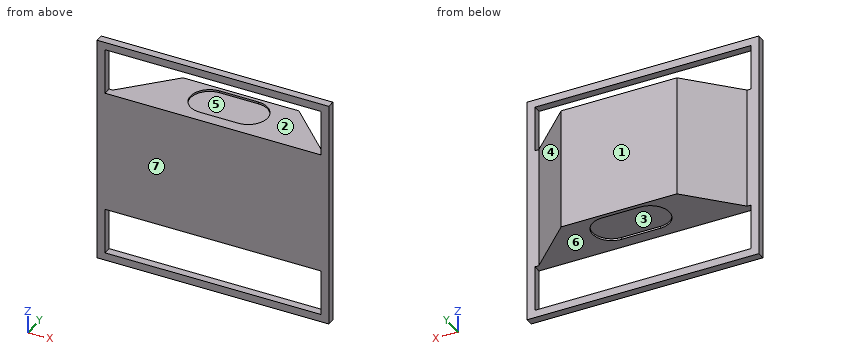
from build123d import *

# Parameters (mm, degrees)
SKETCH_1_W          = 600
SKETCH_1_H          = 600
SKETCH_1_W_2        = 560
SKETCH_1_H_2        = 120
EXTRUDE_1_DEPTH     = 20
EXTRUDE_2_DEPTH     = 320
CUT_EXTRUDE_1_DEPTH = 5
CUT_EXTRUDE_START   = -320
CUT_EXTRUDE_3_DEPTH = 5


with BuildPart() as part:
    # 草图1 → 凸台-拉伸1 (new body)
    with BuildSketch(Plane(origin=(0, 0, 0), x_dir=(1, 0, 0), z_dir=(0, 1, 0))):
        Rectangle(SKETCH_1_W, SKETCH_1_H)
        with Locations((0, 220)):
            Rectangle(SKETCH_1_W_2, SKETCH_1_H_2, mode=Mode.SUBTRACT)
        with Locations((0, -220)):
            Rectangle(SKETCH_1_W_2, SKETCH_1_H_2, mode=Mode.SUBTRACT)
    extrude(amount=EXTRUDE_1_DEPTH)

    # 草图2 → 凸台-拉伸2 (add)
    with BuildSketch(Plane.XY.offset(160)):
        Polygon((-270, 20), (-270, 0), (270, 0), (270, 20), (150, 140), (-150, 140), align=None)
    extrude(amount=-EXTRUDE_2_DEPTH)

    # 草图3 → 切除-拉伸1 (cut)
    with BuildSketch(Plane.XY.offset(160)):
        with BuildLine():
            Line((50, 130), (-50, 130))
            ThreePointArc((-50, 130), (-100, 80), (-50, 30))
            Line((-50, 30), (50, 30))
            ThreePointArc((50, 30), (100, 80), (50, 130))
        make_face()
    extrude(amount=-CUT_EXTRUDE_1_DEPTH, mode=Mode.SUBTRACT)

    # 草图3<3> → 切除-拉伸3 (cut)
    with BuildSketch(Plane.XY.offset(160).offset(CUT_EXTRUDE_START)):
        with BuildLine():
            Line((50, 130), (-50, 130))
            ThreePointArc((-50, 130), (-100, 80), (-50, 30))
            Line((-50, 30), (50, 30))
            ThreePointArc((50, 30), (100, 80), (50, 130))
        make_face()
    extrude(amount=CUT_EXTRUDE_3_DEPTH, mode=Mode.SUBTRACT)


solid = part.part
Model file for the job. Use its own axes, mm. Face numbers are marked on the shaded views. A direction names the side the tool comes from. Coordinates: 2 decimals unless noted, no trailing zeros. Loops run counter-clockwise (first coordinate to the right, second up) from the corner with the lowest first, then second, coordinate; pieces in that order, holes last. Notation, with made-up numbers: (20, 28.5) -> (70, 28.5) arc R30 ccw to (70, 56.5) -> close; hole circle Ø1 at (75.25, 85.5). An arc over 180 degrees is marked (long way). Use one line per item in the form item = value. Start each with the question number.
(1) Cut at A-A on x = 177. Give the cut face in (y, z), and give its area (3 significant figures).
(2) Cut at B-B on z = -218. Give the cut face in (x, y).
(3) Pull direction X, two halves, no side cores. Call the marked faces 1, 2, 3 and 4: pulls with the +X half, pulls with the -X half, needs draft (parallel to the pull), parting line crosses it, or undercut.
(4) Tool access for the marked faces 5, 6 and 7: list every direction of +Z, -Z, +X, -X, +Y, -Y with a clear straight run to the whole face (end or side of a thin tool).
(5) Cut at C-C on z = -48.5. Give the cut face in (x, y).
(6) Cut at D-D on x = -252. Give the cut face in (y, z), and give its area (3 significant figures).
(7) Probe probe 1 along Z at (x, y) = (-1.5, 8.5); probe 2 along Z at (x, y) = (-113.5, 58); probe 3 along Z at (x, y) = (-80, 77.5). List the from-to ranges inside material, lowest first. Write a range as from..to.
(8) Flat gauge pins, fed straight in: pin 1 (12 mm diameter, centred on x = -175.5, z = 38, fed in from +Y); pin 2 (5 mm diameter, centred on x = -191, z = 68, fed in from +Y); pin 3 (12 mm diameter, centred on x = 157, y = 65.5, fed in from -Z). Where does each tip first touch, or does it go through?
Values:
q1.outline = (0, -300) -> (20, -300) -> (20, -280) -> (0, -280) -> close; (0, -160) -> (113, -160) -> (113, 160) -> (0, 160) -> close; (0, 280) -> (20, 280) -> (20, 300) -> (0, 300) -> close
q1.area = 37,000 mm2
q2.outline = (-300, 0) -> (-280, 0) -> (-280, 20) -> (-300, 20) -> close; (280, 0) -> (300, 0) -> (300, 20) -> (280, 20) -> close
q3.face_1 = needs draft
q3.face_2 = undercut
q3.face_3 = undercut
q3.face_4 = pulls with the +X half
q4.face_5 = +Z
q4.face_6 = +Y, -Y
q4.face_7 = +Z, -Z, +X, -X, -Y
q5.outline = (-300, 0) -> (300, 0) -> (300, 20) -> (270, 20) -> (150, 140) -> (-150, 140) -> (-270, 20) -> (-300, 20) -> close
q6.outline = (0, -300) -> (20, -300) -> (20, -280) -> (0, -280) -> close; (0, -160) -> (38, -160) -> (38, 160) -> (0, 160) -> close; (0, 280) -> (20, 280) -> (20, 300) -> (0, 300) -> close
q6.area = 13,000 mm2
q7.probe_1 = -300..-280, -160..160, 280..300
q7.probe_2 = -160..160
q7.probe_3 = -155..155
q8.pin_1 = 120.5
q8.pin_2 = 101.5
q8.pin_3 = -160
